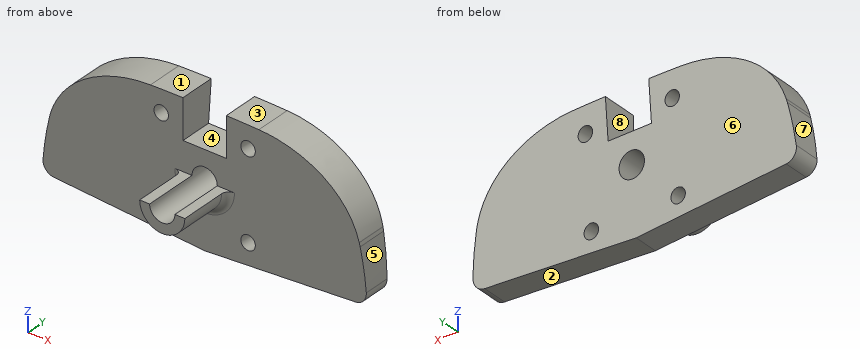
Autodesk Inventor part; units mm, degrees
ref_plane "YZ Plane" through (0, 0, 0) normal (1, 0, 0) x (0, 1, 0)
ref_plane "XZ Plane" through (0, 0, 0) normal (0, 1, 0) x (-1, 0, 0)
ref_plane "XY Plane" through (0, 0, 0) normal (0, 0, 1) x (1, 0, 0)
sketch "Skizze1" plane through (0, 0, 0) normal (0, 1, 0) x (-1, 0, 0)
  line L0 (0, -18.5) -> (0, 18.5) construction
  arc A0 (41.721, -15.6557) -> (44.7394, -12.1512) centre (41.5, -12.4133) ccw
  arc A1 (-44.7394, -12.1512) -> (-41.721, -15.6557) centre (-41.5, -12.4133) ccw
  line L1 (0, -18.5) -> (-41.721, -15.6557)
  line L2 (0, -18.5) -> (41.721, -15.6557)
  line L3 (65.5763, 0) -> (-65.5763, 0)
  line L4 (-6, 7.5) -> (6, 7.5)
  line L5 (6, 7.5) -> (6, 18.5)
  line L6 (6, 18.5) -> (-6, 18.5) construction
  line L7 (-6, 18.5) -> (-6, 7.5)
  line L8 (-6, 7.5) -> (6, 18.5) construction
  line L9 (6, 7.5) -> (-6, 18.5) construction
  arc A2 (-43.0393, -1) -> (-44.7394, -12.1512) centre (35, -18.603) ccw
  spline S0 degree 3 poles (-43.0393, -1) (-40.2103, 11.542) (-27.2639, 17.9936) (-15, 18.3281) knots 0 0 0 0 1 1 1 1
  arc A3 (44.7394, -12.1512) -> (43.0393, -1) centre (-35, -18.603) ccw
  spline S1 degree 3 poles (15, 18.3281) (27.2639, 17.9936) (40.2103, 11.542) (43.0393, -1) knots 0 0 0 0 1 1 1 1
  arc A4 (15, 18.3281) -> (6, 18.5) centre (0, -531.4673) ccw
  arc A5 (-6, 18.5) -> (-15, 18.3281) centre (0, -531.4673) ccw
  point P0 (0, 0)
  point P1 (0, 0)
  point P2 (0, 13)
  dimension "d3" = 6.5
  dimension "d4" = 3.9
  dimension "d5" = 83
  dimension "d6" = 12
  dimension "d9" = 80
  dimension "d10" = 70
  dimension "d12" = 30
  dimension "d13" = 550
  dimension "d14" = 26
  dimension "d15" = 11
  dimension "d16" = 1
extrude "Extrusion1" add sketch "Skizze1" along normal blind 10
sketch "Skizze2" plane through (0, 10, 0) normal (0, 1, 0) x (1, 0, 0)
  circle A0 centre (0, 0.5) radius 3.5
  line L0 (12.0208, 12.5208) -> (-12.0208, 12.5208) construction
  line L1 (-12.0208, 12.5208) -> (-12.0208, -11.5208) construction
  line L2 (-12.0208, -11.5208) -> (12.0208, -11.5208) construction
  line L3 (12.0208, -11.5208) -> (12.0208, 12.5208) construction
  line L4 (12.0208, 12.5208) -> (-12.0208, -11.5208) construction
  line L5 (-12.0208, 12.5208) -> (12.0208, -11.5208) construction
  line L6 (-12.0208, -11.5208) -> (-6.364, -17.1777) construction
  line L7 (12.0208, 12.5208) -> (17.6777, 6.864) construction
  line L8 (12.0208, -11.5208) -> (6.364, -17.1777) construction
  line L9 (-12.0208, 12.5208) -> (-17.6777, 6.864) construction
  circle A1 centre (12.0208, -11.5208) radius 2
  circle A2 centre (-12.0208, -11.5208) radius 2
  circle A3 centre (-12.0208, 12.5208) radius 2
  circle A4 centre (12.0208, 12.5208) radius 2
  point P0 (0, 18.5)
  point P1 (0, 0)
  dimension "d17" = 7
  dimension "d20" = 18
  dimension "d27" = 8
  dimension "d28" = 8
  dimension "d29" = 8
  dimension "d30" = 8
  dimension "d31" = 34
  dimension "d32" = 4
  dimension "d33" = 34
  dimension "d34" = 45
extrude "Extrusion2" cut sketch "Skizze2" against normal up to next contours A0
sketch "Skizze3" plane through (0, 0, 0) normal (0, -1, 0) x (1, 0, 0)
  circle A0 centre (0, -0.5) radius 3.5
  arc A1 (-6.25, -0.5) -> (6.25, -0.5) centre (0, -0.5) ccw
  line L0 (-6.25, -0.5) -> (-3.5, -0.5)
  circle A2 centre (0, -0.5) radius 3.5
  line L1 (3.5, -0.5) -> (6.25, -0.5)
  point P0 (0, 0)
  dimension "d21" = 12.5
extrude "Extrusion3" add sketch "Skizze3" along normal blind 15 contours L1 A1 L0 A0
fillet "Rundung1" radius 2 1 edges at (0, 0, -6.75)
sketch "Skizze5" plane through (0, 0, 0) normal (1, 0, 0) x (0, 1, 0)
  line L0 (10, 18.5) -> (6.7629, -18.5)
  line L1 (6.7629, -18.5) -> (10, -18.5)
  line L2 (10, -18.5) -> (10, 18.5)
  line L3 (10, 3) -> (10, -4)
  line L4 (10, -15.6557) -> (10, -18.5)
  line L5 (10, -18.5) -> (10, -15.6557)
  line L6 (10, -15.6557) -> (10, -12.1512)
  line L7 (10, -12.1512) -> (10, -1)
  line L8 (10, -1) -> (10, 18.3281)
  line L9 (10, 18.3281) -> (10, 18.5)
  line L10 (10, 18.5) -> (10, 7.5)
  line L11 (10, 7.5) -> (10, 18.5)
  line L12 (10, 18.5) -> (10, 18.3281)
  line L13 (10, 18.3281) -> (10, -1)
  line L14 (10, -1) -> (10, -12.1512)
  line L15 (10, -12.1512) -> (10, -15.6557)
  point P0 (0, 0)
  dimension "d35" = 5
extrude "Extrusion4" cut sketch "Skizze5" along normal through all both and the other way through all
sketch "Skizze6" plane through (-6, 9.0376, 7.5) normal (0, 0.9962, -0.0872) x (1, 0, 0)
  line L0 (18.0208, 20.0514) -> (-6.0208, 20.0514) construction
  line L1 (-6.0208, 20.0514) -> (-6.0208, -3.9903) construction
  line L2 (-6.0208, -3.9903) -> (18.0208, -3.9903) construction
  line L3 (18.0208, -3.9903) -> (18.0208, 20.0514) construction
  ellipse E0 centre (6, 8.0306) end of major axis (6, 11.5439) minor radius 3.5
  line L4 (18.0208, 20.0514) -> (-6.0208, -3.9903) construction
  line L5 (-6.0208, 20.0514) -> (18.0208, -3.9903) construction
  line L6 (-6.0208, -3.9903) -> (-2.4853, -7.5258) construction
  line L7 (18.0208, 20.0514) -> (21.5563, 16.5158) construction
  circle A0 centre (18.0208, -3.9903) radius 2
  circle A1 centre (-6.0208, -3.9903) radius 2
  circle A2 centre (-6.0208, 20.0514) radius 2
  circle A3 centre (18.0208, 20.0514) radius 2
  point P0 (6, 8.2591)
  dimension "d38" = 45
  dimension "d39" = 5
  dimension "d40" = 5
  dimension "d41" = 34
  dimension "d42" = 4
extrude "Extrusion5" cut sketch "Skizze6" against normal blind 10 contours A0 | A1 | A2 | A3
equation "\"G_L\" = 0"
equation "\"G_H\" = 0"
equation "\"G_B\" = 0"
properties part number "Motormount_5grad" material "GEDA Stahl"
Geometry: final body of the model. Coordinates: model frame, mm. Face numbers are marked on the shaded views. A direction names the side the tool comes from. Give positions to 0.01 mm unless a question says otherwise; leave off trailing zeros. Loops run counter-clockwise (first coordinate to the right, second up) from the corner with the lowest first, then second, coordinate; pieces in that order, holes last. Notation, with made-up numbers: (70, 44.5) -> (109, 44.5) arc R18 ccw to (109, 67.5) -> close; hole circle Ø8 at (20.5, -27). An arc over 180 degrees is marked (long way). Put each result on its own line as item: value.
1. Cut plane A-A (y = -12.75). Return the cut outline in (x, z), plus the area to 3 significant figures.
Taken from the geometry:
outline: (-6.25, -0.5) arc R6.25 ccw to (6.25, -0.5) -> (3.5, -0.5) arc R3.5 cw to (-3.5, -0.5) -> close
area: 42.1 mm2
2. Pull-direction query (X, two-part tool) for the marked faces 5, 6, 7 and 8; classes: released by +X, released by -X, zero draft, split by the parting line, or undercut.
Taken from the geometry:
face 5: released by +X
face 6: zero draft
face 7: released by -X
face 8: undercut
3. Cut plane B-B (y = 2.75). Count the separate pieces of the cut face and the enclosed holes in it, plus the area to 3 significant figures.
Taken from the geometry:
separate pieces: 1
enclosed holes: 5
area: 2,580 mm2
4. Pin query (flat end, axial travel): P1, Ø3, axis at y = 6.5, z = 15.5, coming from the +X side; P2, Ø12, axis at x = -18.5, z = -11, coming from the +Y side; P3, Ø1, axis at y = 7.5, z = 6.5, coming from the -X side; P4, Ø10, axis at y = 6.5, z = -8.5, coming from the +X side. Return the tip coordinate at first contact, or that it passes through.
Taken from the geometry:
P1: stops at x = 31.28
P2: stops at y = 7.94
P3: stops at x = -40.08
P4: stops at x = 44.75
5. Set-up query: the marked faces 1, 2, 3 and 4. Return all of +Z, -Z, +X, -X, +Y, -Y with unobstructed straight access to the full face (end or side cutting, diameter ignored); none if empty.
Taken from the geometry:
face 1: +Z, -X, +Y, -Y
face 2: -Z, +X, +Y, -Y
face 3: +Z, +X, +Y, -Y
face 4: +Z, +Y, -Y
6. Ray query, line 1 along Z through (x, y) = (1, 5); line 2 along Z through (x, y) = (0, 3.75); line 3 along X through (y, z) = (6.25, 2). Return the intervals inside material, ascending. Write a range as [from, to].
Taken from the geometry:
line 1: z = [-18.43, -3.85], [2.85, 7.5]
line 2: z = [-18.5, -4], [3, 7.5]
line 3: x = [-42.13, -2.45], [2.45, 42.13]
